from build123d import *

# Parameters (mm, degrees)
EXTRUDE_1_DEPTH          = 108
CHAMFER_1_SIZE           = 55
CHAMFER_1_SIZE2          = 5
CHAMFER_2_SIZE           = 5
CHAMFER_2_SIZE2          = 55
CHAMFER_3_SIZE           = 4
SKETCH_2_R               = 42.5
CUT_EXTRUDE_1_DEPTH      = 108
SKETCH_3_R               = 45
CUT_EXTRUDE_2_DEPTH      = 11
CUT_EXTRUDE_START        = -97
SKETCH_3_2_R             = 45
CUT_EXTRUDE_3_DEPTH      = 11
SKETCH_4_R               = 5
CUT_EXTRUDE_4_DEPTH      = 21
SKETCH_8_R               = 47.5
CUT_EXTRUDE_5_DEPTH      = 2
CUT_EXTRUDE_6_REACH      = 165.673
CUT_EXTRUDE_6_END_RADIUS = 42.5
SKETCH_9_R               = 42.5
CHAMFER_4_SIZE           = 1


with BuildPart() as part:
    # 草图1 → 凸台-拉伸1 (new body)
    with BuildSketch(Plane(origin=(0, 0, 0), x_dir=(1, 0, 0), z_dir=(0, 1, 0))):
        with BuildLine():
            Line((-55, 0), (55, 0))
            Line((55, 0), (55, 57))
            ThreePointArc((55, 57), (0, 112), (-55, 57))
            Line((-55, 57), (-55, 0))
        make_face()
    extrude(amount=EXTRUDE_1_DEPTH)

    # 倒角1
    chamfer_1_edges = [part.edges().sort_by_distance(p)[0] for p in [
        (-55, 54, 0),
    ]]
    chamfer_1_side = [part.faces().sort_by_distance(p)[0] for p in [
        (-55, 54, -28.5),
    ]]
    chamfer(chamfer_1_edges, length=CHAMFER_1_SIZE, length2=CHAMFER_1_SIZE2, reference=chamfer_1_side[0])

    # 倒角2
    chamfer_2_edges = [part.edges().sort_by_distance(p)[0] for p in [
        (55, 54, 0),
    ]]
    chamfer_2_side = [part.faces().sort_by_distance(p)[0] for p in [
        (2.5, 54, 0),
    ]]
    chamfer(chamfer_2_edges, length=CHAMFER_2_SIZE, length2=CHAMFER_2_SIZE2, reference=chamfer_2_side[0])

    # 倒角3
    # the kernel refuses this chamfer: 4 mm, written as the material it takes off along each edge
    with BuildSketch(Plane(origin=(-55, 108, -57), x_dir=(-0.027495876610585647, -0.9996219169112968, 0), z_dir=(0, 0, 1)), Plane(origin=(55, 0, -44.713268048), x_dir=(-0.9996219169112968, -0.02749587661058639, 0), z_dir=(0, 0, -1)), Plane(origin=(55, 108, -44.713268048), x_dir=(0.027495876610585647, -0.9996219169112968, 0), z_dir=(0, 0, -1)), Plane(origin=(-55, 0, -57), x_dir=(0.9996219169112968, -0.02749587661058639, 0), z_dir=(0, 0, 1))) as chamfer_3_piece_1:
        Polygon((CHAMFER_3_SIZE * 0.999621916911, CHAMFER_3_SIZE * 0.0274958766106), (-CHAMFER_3_SIZE * 0.0274958766106, CHAMFER_3_SIZE * 0.999621916911), (0, 0), align=None)
    extrude(amount=12.286731952, mode=Mode.SUBTRACT)
    with BuildSketch(Plane(origin=(-60.286731952, 0, 0), x_dir=(0, -0.027495876610586372, -0.9996219169112968), z_dir=(1, 0, 0)), Plane(origin=(-60.286731952, 108, 0), x_dir=(0, -0.9996219169112968, 0.02749587661058639), z_dir=(1, 0, 0))) as chamfer_3_piece_2:
        Polygon((CHAMFER_3_SIZE * 0.999621916911, CHAMFER_3_SIZE * 0.0274958766106), (-CHAMFER_3_SIZE * 0.0274958766106, CHAMFER_3_SIZE * 0.999621916911), (0, 0), align=None)
    extrude(amount=120.573463904, mode=Mode.SUBTRACT)
    with BuildSketch(Plane(origin=(-55.931316952, 0, -65.244486468), x_dir=(0.995516676088184, -0.027495876610586417, -0.09050151600801698), z_dir=(0.09053574604251878, 0, 0.9958932064677039)), Plane(origin=(-55.931316952, 108, -65.244486468), x_dir=(-0.027382956722356327, -0.9996219169112968, 0.0024893597020324005), z_dir=(0.09053574604251878, 0, 0.9958932064677039)), Plane(origin=(49.068683048, 0, 10.244486468), x_dir=(-0.995516676088184, -0.027495876610586358, -0.09050151600801698), z_dir=(0.09053574604251878, 0, -0.9958932064677039)), Plane(origin=(49.068683048, 108, 10.244486468), x_dir=(0.027382956722356445, -0.9996219169112968, 0.0024893597020324114), z_dir=(0.09053574604251878, 0, -0.9958932064677039))) as chamfer_3_piece_3:
        Polygon((CHAMFER_3_SIZE * 0.999621916911, CHAMFER_3_SIZE * 0.0274958766106), (-CHAMFER_3_SIZE * 0.0274958766106, CHAMFER_3_SIZE * 0.999621916911), (0, 0), align=None)
    extrude(amount=75.80026899, mode=Mode.SUBTRACT)
    with BuildSketch(Plane(origin=(0, 0, -57), x_dir=(1, 0, 0), z_dir=(0, 0, 1))) as chamfer_3_piece_4:
        Polygon((55 - CHAMFER_3_SIZE, 0), (55, CHAMFER_3_SIZE), (55, 0), align=None)
    revolve(axis=Axis((0, 0, -57), (0, 1, 0)), revolution_arc=180, mode=Mode.SUBTRACT)
    with BuildSketch(Plane(origin=(0, 108, -57), x_dir=(1, 0, 0), z_dir=(0, 0, 1))) as chamfer_3_piece_5:
        Polygon((55, -CHAMFER_3_SIZE), (55 - CHAMFER_3_SIZE, 0), (55, 0), align=None)
    revolve(axis=Axis((0, 108, -57), (0, 1, 0)), revolution_arc=180, mode=Mode.SUBTRACT)

    # 草图2 → 切除-拉伸1 (cut)
    with BuildSketch(Plane(origin=(0, 108, 0), x_dir=(1, 0, 0), z_dir=(0, 1, 0))):
        with Locations(Location((0, 57, 0), (0, 0, 270))):
            Circle(SKETCH_2_R)
    extrude(amount=-CUT_EXTRUDE_1_DEPTH, mode=Mode.SUBTRACT)

    # 草图3 → 切除-拉伸2 (cut)
    with BuildSketch(Plane(origin=(0, 108, 0), x_dir=(1, 0, 0), z_dir=(0, 1, 0))):
        with Locations(Location((0, 57, 0), (0, 0, 270))):
            Circle(SKETCH_3_R)
    extrude(amount=-CUT_EXTRUDE_2_DEPTH, mode=Mode.SUBTRACT)

    # 草图3<2> → 切除-拉伸3 (cut)
    with BuildSketch(Plane(origin=(0, 108, 0), x_dir=(1, 0, 0), z_dir=(0, 1, 0)).offset(CUT_EXTRUDE_START)):
        with Locations(Location((0, 57, 0), (0, 0, 270))):
            Circle(SKETCH_3_2_R)
    extrude(amount=-CUT_EXTRUDE_3_DEPTH, mode=Mode.SUBTRACT)

    # 草图4 → 切除-拉伸4 (cut)
    with BuildSketch(Plane.XY):
        with Locations((40, 94)):
            Circle(SKETCH_4_R)
        with Locations((40, 14)):
            Circle(SKETCH_4_R)
        with Locations((-40, 14)):
            Circle(SKETCH_4_R)
        with Locations((-40, 94)):
            Circle(SKETCH_4_R)
    extrude(amount=-CUT_EXTRUDE_4_DEPTH, mode=Mode.SUBTRACT)

    # 草图6 → 切除-旋转1 (revolve, cut)
    with BuildSketch(Plane(origin=(0, 19, 0), x_dir=(-1, 0, 0), z_dir=(0, -1, 0))):
        Polygon((55, 57), (55, 52), (45, 52), (45, 55), (35, 55), (35, 57), align=None)
    revolve(axis=Axis((-55, 19, -57), (1, 0, 0)), mode=Mode.SUBTRACT)

    # 草图7 → 切除-旋转2 (revolve, cut)
    with BuildSketch(Plane(origin=(0, 39, 0), x_dir=(-1, 0, 0), z_dir=(0, -1, 0))):
        Polygon((35, 55), (35, 57), (55, 57), (55, 52), (45, 52), (45, 55), align=None)
    revolve(axis=Axis((-55, 39, -57), (1, 0, 0)), mode=Mode.SUBTRACT)

    # 草图8 → 切除-拉伸5 (cut)
    with BuildSketch(Plane.XY):
        with Locations((0, 54)):
            Circle(SKETCH_8_R)
    extrude(amount=-CUT_EXTRUDE_5_DEPTH, mode=Mode.SUBTRACT)

    # 切除-拉伸6: up to this cylinder (the profile starts outside it)
    cut_extrude_6_end = Plane(origin=(0, 54, -57), z_dir=(0, 1, 0)) * Cylinder(CUT_EXTRUDE_6_END_RADIUS, 417.346, mode=Mode.PRIVATE)
    # 草图9 → 切除-拉伸6 (cut, up to the surface)
    with BuildSketch(Plane.XY.offset(-2), mode=Mode.PRIVATE) as cut_extrude_6_sk1:
        with Locations((0, 54)):
            Circle(SKETCH_9_R)
    cut_extrude_6_tool1 = extrude(cut_extrude_6_sk1.sketch, amount=-CUT_EXTRUDE_6_REACH, mode=Mode.PRIVATE) - cut_extrude_6_end
    add(cut_extrude_6_tool1.solids().sort_by_distance((0, 54, -2))[0], mode=Mode.SUBTRACT)

    # 倒角4
    chamfer_4_edges = [part.edges().sort_by_distance(p)[0] for p in [
        (-42.5, 54, -2),
    ]]
    chamfer(chamfer_4_edges, length=CHAMFER_4_SIZE)


solid = part.part
Geometry: final body of the model. Coordinates: model frame, mm. A direction names the side the tool comes from. Give positions to 0.01 mm unless a question says otherwise; leave off trailing zeros. Write each loop counter-clockwise with the first axis right and the second up, starting at its lowest first coordinate (ties: lowest second). Pieces come first, ordered by that corner, then holes. Notation, with made-up numbers: (-11.5, -23) - (30.5, -23) arc R26 ccw to (30.5, 3) - close; hole circle Ø8 at (64, 89). An arc over 180 degrees is marked (long way). Return JSON: item names as keys, results as strings. Group by question number.
1) Section B-B on z = -28. Return the cut outline in (x, y), plus the area to 3 significant figures.
2) Section A-A on x = 0. State how many separate pieces and enclosed holes the cut face has, plus the area to 3 significant figures.
3) First-contact query: P1, Ø4, axis at y = 37.5, z = -44, coming from the +X side; P2, Ø11, axis at x = -39.5, y = 92, coming from the +Z side; P3, Ø6, axis at x = -40, y = 94, coming from the -Z side; P4, Ø6, axis at y = 22, z = -69, coming from the -X side. Flat tips, straight axial feed; report the tip coordinate or a pass-through.
4) Section C-C on y = 54. Return the cut outline in (x, z).
5) Set-up query: faces 5 (the cylindrical face through (1.87, 54.6, -99.46)), 6 (the cylindrical face through (-50, 36, -61)), 7 (the cylindrical face through (-45, 94, -10)), 8 (the flat face through (26.9, 11, -23.9)), 9 (the flat face through (0, 0, -10)). Return all of +Z, -Z, +X, -X, +Y, -Y with unobstructed straight access to the full face (end or side cutting, diameter ignored); none if empty.
6) Mould query, pull axis Z, two halves, no side actions, for faces 1 (the flat face through (-52.465, 53.3, -27.115)), 2 (the cylindrical face through (-43.708, 40.774, -56.077)), 3 (the flat face through (53, 2, -56)), 4 (the cylindrical face through (-17.235, 5.577, -15.431)). Classes: released by +Z, released by -Z, zero draft, split by the parting line, or undercut.
7) Line query: line 1 (X direction, y = 47.5, z = -57.5); line 2 (Y direction, x = -49.5, z = -57); line 3 (X direction, y = 103.25, z = -57). Output: solid intervals per line, ascending.
Filled in:
{
 "1": {"outline": "(-52.55, 4) - (-48.53, 0) - (-34.41, 0) - (-34.41, 11) - (-31.07, 11) - (-31.07, 25) arc R42.5 cw to (-31.07, 83) - (-31.07, 97) - (-34.41, 97) - (-34.41, 108) - (-48.53, 108) - (-52.55, 104) - close; (31.07, 11) - (34.41, 11) - (34.41, 0) - (48.53, 0) - (52.55, 4) - (52.55, 104) - (48.53, 108) - (34.41, 108) - (34.41, 97) - (31.07, 97) - (31.07, 83) arc R42.5 cw to (31.07, 25) - close", "area": "3,550 mm^2"},
 "2": {"separate pieces": "3", "enclosed holes": "0", "area": "1,520 mm^2"},
 "3": {"P1": "stops at x = 54.18", "P2": "stops at z = 0", "P3": "stops at z = -97.69", "P4": "stops at x = -54.26"},
 "4": {"outline": "(-55, -57) arc R55 ccw to (55, -57) - (55, -55) - (50, 0) - (47.5, 0) - (47.5, -2) - (43.5, -2) - (42.5, -3) - (42.5, -57) arc R42.5 cw to (-42.5, -57) - (-42.5, -3) - (-43.5, -2) - (-47.5, -2) - (-47.5, 0) - (-50, 0) - (-55, -55) - close"},
 "5": {"face 5": "+Y, -Y", "face 6": "-X", "face 7": "+Z", "face 8": "-Y", "face 9": "+Z, -Z, +X, -X, -Y"},
 "6": {"face 1": "released by +Z", "face 2": "undercut", "face 3": "zero draft", "face 4": "undercut"},
 "7": {"line 1": "x = -55 to -42.5, 42.5 to 55", "line 2": "y = 0 to 14, 24 to 34, 44 to 108", "line 3": "x = -55 to -45, 45 to 55"}
}
